Here's the drawing with two shaded views (mm, measured from the low corner). I have some questions. A direction names the side the tool comes from. Coordinates: 2 decimals unless noted, no trailing zeros. Write each loop counter-clockwise with the first axis right and the second up, starting at its lowest first coordinate (ties: lowest second). Pieces come first, ordered by that corner, then holes. Notation, with made-up numbers: (55, 43.25) -> (66, 43.25) arc R26 ccw to (66, 77.25) -> close; hole circle Ø7 at (-18.5, -10). An arc over 180 degrees is marked (long way). Put each result on its own line as item: value. Start each with the question number.
Item 1: If we mould it in two halves opening along Z, with no side actions, what happens to the marked faces 1, 2 and 3? For each: released by +Z, released by -Z, zero draft, split by the parting line, or undercut.
Item 2: I want a section at B-B, the plane x = 412. List the corners of the cut face in (y, z) for me, then the cut area to 3 significant figures.
Item 3: On a 3-axis mill with a long thin cutter (end or side, diameter ignored), from which of +Z, -Z, +X, -X, +Y, -Y can I reach the whole of each face in a straight line? I mean the marked faces 4, 5, 6, 7 and 8. Say none if no direction works.
Item 4: For pin 1 (10 mm diameter, centred on x = 833, z = 540.5, fed in from +Y); pin 2 (6 mm diameter, centred on y = 717.5, z = 590, fed in from -X); pin 3 (3 mm diameter, centred on x = 176, y = 111.5, fed in from -Z), each with a flat end and sliding along its axis, tell me the tip position at first contact or that it passes through.
Item 5: I want a section at A-A, the plane y = 869.5. List the corners of the cut face in (x, z) for me.
Item 6: I need wall thicknesses on line 1 (Z direction, x = 369, y = 138); line 2 (Y direction, x = 294.5, z = 944); line 3 (X direction, y = 697.5, z = 434.5). Which ranges of each line are inside material? Lowest first, please. Write a range as [from, to].
Item 7: I want a section at C-C, the plane z = 951.5. List the corners of the cut face in (x, y) for me, then the cut area to 3 significant figures.
Item 8: I want a section at D-D, the plane z = 440. List the corners of the cut face in (x, y) for me, then the cut area to 3 significant figures.
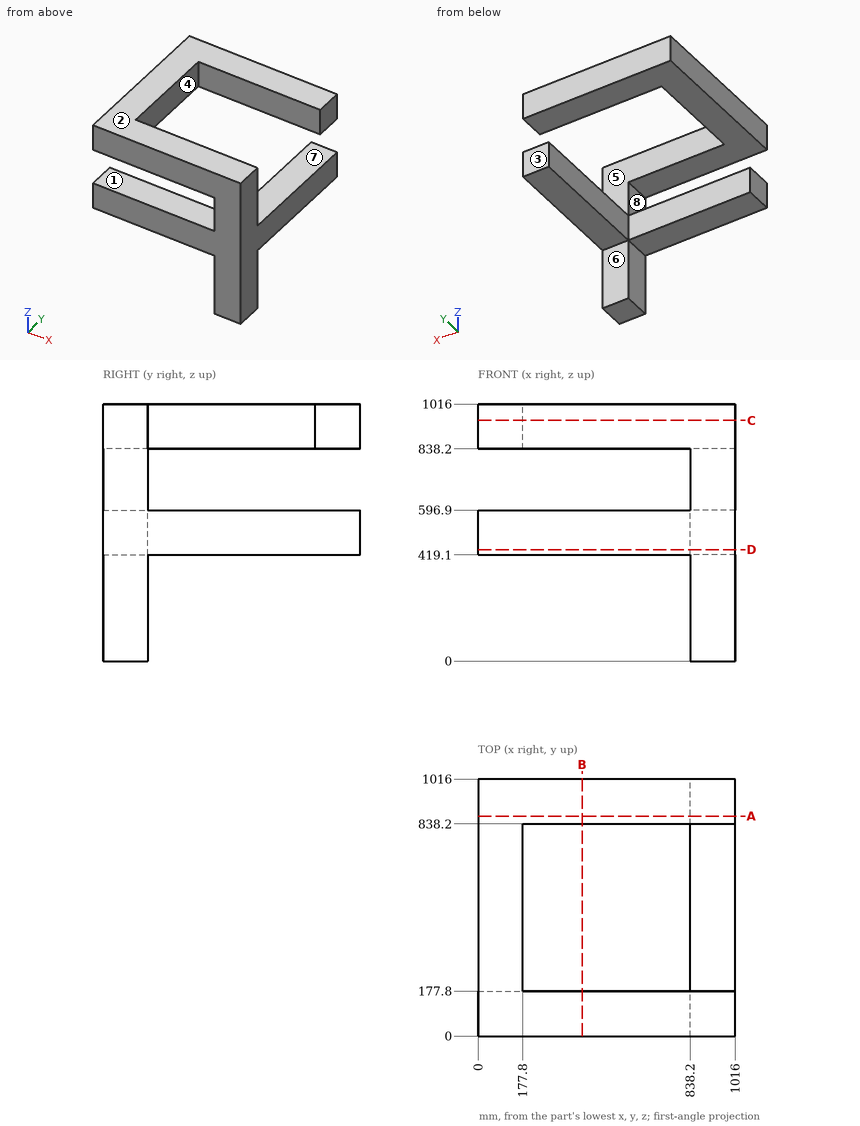
Calculated:
1. face 1: undercut
1. face 2: released by +Z
1. face 3: zero draft
2. outline: (0, 419.1) -> (177.8, 419.1) -> (177.8, 596.9) -> (0, 596.9) -> close; (0, 838.2) -> (177.8, 838.2) -> (177.8, 1016) -> (0, 1016) -> close; (838.2, 838.2) -> (1016, 838.2) -> (1016, 1016) -> (838.2, 1016) -> close
2. area: 94,800 mm2
3. face 4: +Z, -Z, +X
3. face 5: +Z, +X
3. face 6: -Z, +X, -X, +Y
3. face 7: +X, -X, +Y
3. face 8: -X, +Y, -Y
4. pin 1: stops at y = 177.8
4. pin 2: stops at x = 838.2
4. pin 3: stops at z = 419.1
5. outline: (0, 838.2) -> (1016, 838.2) -> (1016, 1016) -> (0, 1016) -> close; (838.2, 419.1) -> (1016, 419.1) -> (1016, 596.9) -> (838.2, 596.9) -> close
6. line 1: z = [419.1, 596.9], [838.2, 1016]
6. line 2: y = [0, 177.8], [838.2, 1016]
6. line 3: x = [838.2, 1016]
7. outline: (0, 0) -> (1016, 0) -> (1016, 177.8) -> (177.8, 177.8) -> (177.8, 838.2) -> (1016, 838.2) -> (1016, 1016) -> (0, 1016) -> close
7. area: 479,000 mm2
8. outline: (0, 0) -> (1016, 0) -> (1016, 1016) -> (838.2, 1016) -> (838.2, 177.8) -> (0, 177.8) -> close
8. area: 330,000 mm2
